Read the model definition and answer for the solid it produces. Units are mm, in the model's axes. Face numbers are marked on the shaded views. A direction names the side the tool comes from. Coordinates: 2 decimals unless noted, no trailing zeros. Write each loop counter-clockwise with the first axis right and the second up, starting at its lowest first coordinate (ties: lowest second). Pieces come first, ordered by that corner, then holes. Notation, with made-up numbers: (-6.75, 33) -> (16.25, 33) arc R22 ccw to (16.25, 55) -> close; hole circle Ø10 at (76.25, 32). An arc over 180 degrees is marked (long way). Write item = value, one per line. Start each with the question number.
1) Flat-ended cylindrical pins translate along their axes: pin 1 Ø1.5 at (y, z) = (27.5, 27.5) entering from +X; pin 2 Ø4 at (y, z) = (23.5, 38) entering from -X; pin 3 Ø3 at (y, z) = (5, 48) entering from -X. Find the tip coordinate at first contact, or state that the pin passes through.
2) For a pull along X with two mould halves and no side action, classify the marked faces 1, 2 and 3 as released by +X, released by -X, zero draft, split by the parting line, or undercut.
3) Find the intervals of material crossed by line 1 along Z through (x, y) = (64.5, 20.5); line 2 along Z through (x, y) = (55.5, 2); line 3 along X through (y, z) = (28, 54), in increasing order. Write a range as from..to.
4) Section A-A (x = 64) is taken. Determine the outline of the cut face in (y, z).
5) Section C-C (y = 23) is taken. Determine the outline of the cut face in (x, z).
6) A tool of negligible diameter and unlimited length cuts with its end or side. For the marked faces 4 and 5, from which of +Z, -Z, +X, -X, +Y, -Y can it reach the whole face along a straight path? Write none if from no direction.
7) Section B-B (z = 30) is taken. Determine the outline of the cut face in (x, y).
8) Section D-D (x = 6) is taken. Determine the outline of the cut face in (y, z).
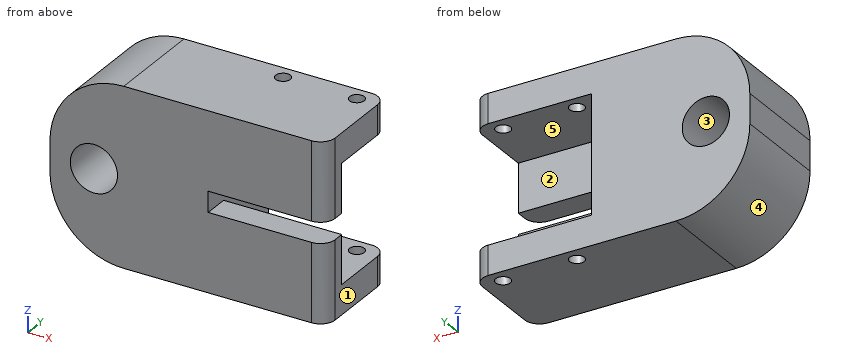
from build123d import *

# Parameters (mm, degrees)
SKETCH1_W                  = 93.6
SKETCH1_H                  = 33.62
BOSS_EXTRUDE2_DEPTH        = 60
CUT_EXTRUDE2_DEPTH         = 40
FILLET2_R                  = 25
F_16_0_16_DIAMETER_HOLE2_D = 16
FILLET3_R                  = 5
SKETCH13_W                 = 40
SKETCH13_H                 = 7
CUT_EXTRUDE3_DEPTH         = 103.58979849
F_5_0_5_DIAMETER_HOLE1_D   = 5


with BuildPart() as part:
    # Sketch1 → Boss-Extrude2 (new body)
    with BuildSketch(Plane.XY):
        with Locations((32.570440053, 16.81)):
            Rectangle(SKETCH1_W, SKETCH1_H)
    extrude(amount=BOSS_EXTRUDE2_DEPTH)

    # Sketch8 → Cut-Extrude2 (cut)
    with BuildSketch(Plane(origin=(79.370440053, 0, 0), x_dir=(0, 0, -1), z_dir=(1, 0, 0))):
        Polygon((-30, 8.62), (-10, 8.62), (-10, 33.62), (-50, 33.62), (-50, 8.62), align=None)
    extrude(amount=-CUT_EXTRUDE2_DEPTH, mode=Mode.SUBTRACT)

    # Fillet2
    fillet2_edges = [part.edges().sort_by_distance(p)[0] for p in [
        (-14.229559947, 16.81, 60),
        (-14.229559947, 16.81, 0),
    ]]
    fillet(fillet2_edges, radius=FILLET2_R)

    # Ø16.0 (16) Diameter Hole2 (through all)
    with Locations(Plane(origin=(0.670440053, 33.62, 30), x_dir=(1, 0, 0), z_dir=(0, 1, 0))):
        with Locations((0, 0)):
            Hole(F_16_0_16_DIAMETER_HOLE2_D / 2)

    # Fillet3
    fillet3_edges = [part.edges().sort_by_distance(p)[0] for p in [
        (79.370440053, 33.62, 5),
        (79.370440053, 33.62, 55),
        (79.370440053, 0, 30),
    ]]
    fillet(fillet3_edges, radius=FILLET3_R)

    # Sketch13 → Cut-Extrude3 (cut, through all)
    with BuildSketch(Plane(origin=(0, 8.62, 0), x_dir=(1, 0, 0), z_dir=(0, 1, 0))):
        with Locations((59.370440053, -30)):
            Rectangle(SKETCH13_W, SKETCH13_H)
    extrude(amount=-CUT_EXTRUDE3_DEPTH, mode=Mode.SUBTRACT)

    # Ø5.0 (5) Diameter Hole1 (through all)
    with Locations(Plane(origin=(72.370440053, 28.62, 60), x_dir=(1, 0, 0), z_dir=(0, 0, 1))):
        with Locations((0, 0), (-25, 0)):
            Hole(F_5_0_5_DIAMETER_HOLE1_D / 2)


solid = part.part
Answer key:
q1.pin_1 = 39.37
q1.pin_2 = -14.21
q1.pin_3 = -11.43
q2.face_1 = released by +X
q2.face_2 = zero draft
q2.face_3 = undercut
q3.line_1 = 0..10, 50..60
q3.line_2 = 0..26.5, 33.5..60
q3.line_3 = -5.48..44.95, 49.79..69.95, 74.79..79.37
q4.outline = (0, 0) -> (33.62, 0) -> (33.62, 10) -> (8.62, 10) -> (8.62, 26.5) -> (0, 26.5) -> close; (0, 33.5) -> (8.62, 33.5) -> (8.62, 50) -> (33.62, 50) -> (33.62, 60) -> (0, 60) -> close
q5.outline = (-14.23, 25) arc R25 ccw to (10.77, 0) -> (79.37, 0) -> (79.37, 10) -> (39.37, 10) -> (39.37, 50) -> (79.37, 50) -> (79.37, 60) -> (10.77, 60) arc R25 ccw to (-14.23, 35) -> close; hole circle Ø16 at (0.67, 30)
q6.face_4 = -Z, -X, +Y, -Y
q6.face_5 = +X, +Y
q7.outline = (-14.23, 0) -> (-7.33, 0) -> (-7.33, 33.62) -> (-14.23, 33.62) -> close; (8.67, 0) -> (39.37, 0) -> (39.37, 33.62) -> (8.67, 33.62) -> close
q8.outline = (0, 0.46) -> (33.62, 0.46) -> (33.62, 24.03) -> (0, 24.03) -> close; (0, 35.97) -> (33.62, 35.97) -> (33.62, 59.54) -> (0, 59.54) -> close
